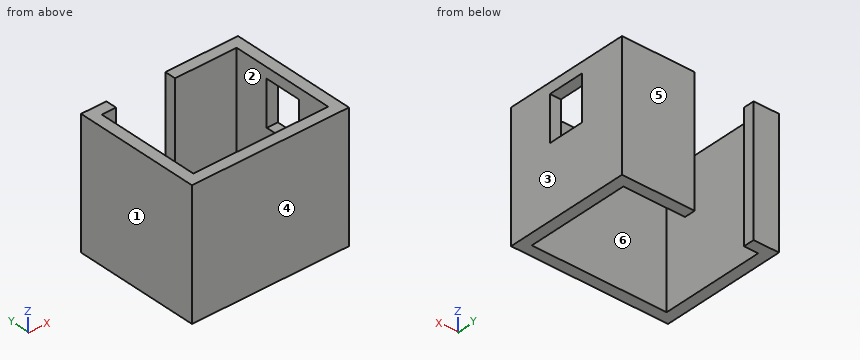
```python
from build123d import *

# Parameters (mm, degrees)
F3_DEPTH   = 240
F5_DEPTH   = 20
F6_W       = 112
F6_H       = 241.106075
F7_DEPTH   = 25
F8_W       = 70.001994
F8_H       = 85
F9_DEPTH   = 25
F10_W      = 50
F10_H      = 198.001994
F11_DEPTH  = 50
F12_DEPTH  = 25
F11_FACE_W = 50
F11_FACE_H = 198.001994
F13_DEPTH  = 70.001


with BuildPart() as f3:
    # F2 (on face) → F3 (new body)
    with BuildSketch(Plane.XY):
        Polygon((-627, -343.001994), (-627, -273), (-627, -187), (-765, -187), (-877, -187), (-925, -187), (-925, -427.001994), (-627, -427.001994), align=None)
        Polygon((-765, -208), (-648, -208), (-648, -273), (-648, -343.001994), (-648, -406.001994), (-904, -406.001994), (-904, -208), (-877, -208), align=None, mode=Mode.SUBTRACT)
    extrude(amount=F3_DEPTH)

    # F4 (on face) → F5 (join)
    with BuildSketch(Plane.XY):
        Polygon((-648, -273), (-648, -208), (-765, -208), (-877, -208), (-904, -208), (-904, -406.001994), (-648, -406.001994), (-648, -343.001994), align=None)
    extrude(amount=F5_DEPTH)

    # F6 (on face) → F7 (cut)
    with BuildSketch(Plane(origin=(0, -187, 0), x_dir=(-1, 0, 0), z_dir=(0, 1, 0))):
        with Locations((821, 140.553037)):
            Rectangle(F6_W, F6_H)
    extrude(amount=-F7_DEPTH, mode=Mode.SUBTRACT)

    # F8 (on face) → F9 (cut)
    with BuildSketch(Plane.YZ.offset(-627)):
        with Locations((-308.000997, 177.5)):
            Rectangle(F8_W, F8_H)
    extrude(amount=-F9_DEPTH, mode=Mode.SUBTRACT)

    # F10 (on face) → F11 (join)
    with BuildSketch(Plane.XY.offset(20)):
        with Locations((-673, -307.000997)):
            Rectangle(F10_W, F10_H)
    extrude(amount=F11_DEPTH)

    # F7_face (on face) → F12 (cut)
    with BuildSketch(Plane(origin=(-777.995456, -302.145343, 20), x_dir=(1, 0, 0), z_dir=(0, 0, 1))):
        Polygon((12.995456, 115.145343), (-99.004544, 115.145343), (-99.004544, 94.145343), (-126.004544, 94.145343), (-126.004544, -103.856651), (79.995456, -103.856651), (79.995456, 94.145343), (12.995456, 94.145343), align=None)
    extrude(amount=-F12_DEPTH, mode=Mode.SUBTRACT)

    # F11_face (on face) → F13 (cut, through all)
    with BuildSketch(Plane(origin=(-673, -307.000997, 70), x_dir=(1, 0, 0), z_dir=(0, 0, 1))):
        Rectangle(F11_FACE_W, F11_FACE_H)
    extrude(amount=-F13_DEPTH, mode=Mode.SUBTRACT)


solid = f3.part
```
Work out the finished part from the listing and answer in its coordinate system (mm). Face numbers are marked on the shaded views. A direction names the side the tool comes from. Coordinates: 2 decimals unless noted, no trailing zeros. Loops run counter-clockwise (first coordinate to the right, second up) from the corner with the lowest first, then second, coordinate; pieces in that order, holes last. Notation, with made-up numbers: (48, 22.5) -> (103, 22.5) arc R28 cw to (103, 48.5) -> close; hole circle Ø3 at (7, -25.75). An arc over 180 degrees is marked (long way). Answer as CSV lines item,"result".
Q1. The part is cut by section D-D on y = -401. Write down the section's boundary in (x, z).
Findings:
outline,"(-925, 0) -> (-904, 0) -> (-904, 240) -> (-925, 240) -> close; (-648, 0) -> (-627, 0) -> (-627, 240) -> (-648, 240) -> close"
Q2. For a pull along X with two mould halves and no side action, classify the marked faces 1, 2, 3 and 4 as +X half, -X half, draft (parallel to the pull), parting line (faces both ways), or undercut.
Findings:
face 1,"-X half"
face 2,"undercut"
face 3,"+X half"
face 4,"draft"
Q3. Find the intervals of material crossed by probe 1 along X at (y, z) = (-296, 27); probe 2 along X at (y, z) = (-205, 216); probe 3 along Y at (x, z) = (-736, 186), in increasing order.
Findings:
probe 1,"x = -925 to -904, -648 to -627"
probe 2,"x = -925 to -877, -765 to -627"
probe 3,"y = -427 to -406, -208 to -187"
Q4. The part is cut by section C-C on y = -283.5. Write down the section's boundary in (x, z).
Findings:
outline,"(-925, 0) -> (-904, 0) -> (-904, 240) -> (-925, 240) -> close; (-648, 0) -> (-627, 0) -> (-627, 135) -> (-648, 135) -> close; (-648, 220) -> (-627, 220) -> (-627, 240) -> (-648, 240) -> close"
Q5. Each of these flat-tipped pins is pushed along its axis until it touches: pin 1 (5 mm diameter, centred on x = -827.5, z = 129.5, fed in from +Y); pin 2 (23 mm diameter, centred on x = -641, y = -291.5, fed in from -Z). Where does it stop, or does it pass through?
Findings:
pin 1,"stops at y = -406"
pin 2,"stops at z = 0"
Q6. The part is cut by section A-A on z = 205. Write down the section's boundary in (x, y).
Findings:
outline,"(-925, -427) -> (-627, -427) -> (-627, -343) -> (-648, -343) -> (-648, -406) -> (-904, -406) -> (-904, -208) -> (-877, -208) -> (-877, -187) -> (-925, -187) -> close; (-765, -208) -> (-648, -208) -> (-648, -273) -> (-627, -273) -> (-627, -187) -> (-765, -187) -> close"
Q7. The part is cut by section B-B on x = -759. Write down the section's boundary in (y, z), and give its area (3 significant figures).
Findings:
outline,"(-427, 0) -> (-406, 0) -> (-406, 240) -> (-427, 240) -> close; (-208, 0) -> (-187, 0) -> (-187, 240) -> (-208, 240) -> close"
area,"10,100 mm²"
Q8. A tool of negligible diameter and unlimited length cuts with its end or side. For the marked faces 5 and 6, from which of +Z, -Z, +X, -X, +Y, -Y can it reach the whole face along a straight path? Write none if from no direction.
Findings:
face 5,"+Z, -Z, +X, -X, +Y"
face 6,"+Z, -Z"
